Source: CAD feature listing. Evaluate the final solid. Frame: model axes, mm. A direction names the side the tool comes from. Give positions to 0.01 mm unless a question says otherwise; leave off trailing zeros. Order: outer loops, then holes, each group sorted by start corner. A loop starts at its lowest first (then second) coordinate and runs counter-clockwise, first axis right, second up. Notation, with made-up numbers: (66.5, 42) -> (94.5, 42) arc R18 ccw to (94.5, 69) -> close; hole circle Ø4 at (-11, 5.5). An arc over 180 degrees is marked (long way). Answer in a Markdown table with one row per item.
```python
from build123d import *

# Parameters (mm, degrees)
SKETCH1_R            = 2.675
BOSS_EXTRUDE6_DEPTH  = 10
BOSS_EXTRUDE8_START  = -21
BOSS_EXTRUDE8_DEPTH  = 21
SKETCH10_R           = 3.5
CUT_EXTRUDE5_DEPTH   = 191.966382811
SKETCH11_R           = 7.125
CUT_EXTRUDE6_DEPTH   = 5
CUT_EXTRUDE7_START   = -5
SKETCH12_R           = 7.125
CUT_EXTRUDE7_DEPTH   = 5
BOSS_EXTRUDE9_DEPTH  = 5
BOSS_EXTRUDE11_DEPTH = 12
BOSS_EXTRUDE13_START = 12
BOSS_EXTRUDE13_DEPTH = 12
SKETCH18_R           = 6.75
CUT_EXTRUDE11_DEPTH  = 1.67
CUT_EXTRUDE13_DEPTH  = 191.966382811
CUT_EXTRUDE14_DEPTH  = 191.966382811
CUT_EXTRUDE10_DEPTH  = 213.509902322
SKETCH26_R           = 2.675
BOSS_EXTRUDE14_DEPTH = 5
SKETCH27_R           = 2.675
BOSS_EXTRUDE15_DEPTH = 5
SKETCH30_R           = 2.675
CUT_EXTRUDE15_DEPTH  = 10
BOSS_EXTRUDE16_START = 1.67
SKETCH31_R           = 6.75
BOSS_EXTRUDE16_DEPTH = 1.67
SKETCH32_R           = 6.75
BOSS_EXTRUDE17_DEPTH = 2
SKETCH34_R           = 6.35
BOSS_EXTRUDE18_DEPTH = 1.5
SKETCH35_R           = 2.675
BOSS_EXTRUDE19_DEPTH = 4
CUT_EXTRUDE16_DEPTH  = 12
CUT_EXTRUDE17_DEPTH  = 12
FILLET1_R            = 10


with BuildPart() as part:
    # Sketch1 → Boss-Extrude6 (new body)
    with BuildSketch(Plane.XY):
        with BuildLine():
            Line((182.426294195, 92.707675116), (186.967804891, 79.877060143))
            ThreePointArc((186.967804891, 79.877060143), (187.827472336, 74.871963218), (186.967804891, 69.866866293))
            Line((186.967804891, 69.866866293), (182.426294195, 57.03625132))
            ThreePointArc((182.426294195, 57.03625132), (179.86789414, 53.655758914), (175.827472336, 52.371963218))
            Line((175.827472336, 52.371963218), (157.827472336, 52.371963218))
            Line((157.827472336, 52.371963218), (157.827472336, 64.371963218))
            Line((157.827472336, 64.371963218), (137.827472336, 64.371963218))
            Line((137.827472336, 64.371963218), (137.827472336, 85.371963218))
            Line((137.827472336, 85.371963218), (157.827472336, 85.371963218))
            Line((157.827472336, 85.371963218), (157.827472336, 97.371963218))
            Line((157.827472336, 97.371963218), (175.827472336, 97.371963218))
            ThreePointArc((175.827472336, 97.371963218), (179.86789414, 96.088167522), (182.426294195, 92.707675116))
        make_face()
        with Locations((155.487472336, 74.871963218)):
            Circle(SKETCH1_R, mode=Mode.SUBTRACT)
    extrude(amount=BOSS_EXTRUDE6_DEPTH)

    # Sketch9 → Boss-Extrude8 (add)
    with BuildSketch(Plane(origin=(0, 85.371963218, 0), x_dir=(1, 0, 0), z_dir=(0, 1, 0)).offset(BOSS_EXTRUDE8_START)):
        with BuildLine():
            Line((137.827472336, 0), (157.827472336, 0))
            ThreePointArc((157.827472336, 0), (154.893165251, 7.076438626), (147.81227561, 9.999988453))
            Line((147.81227561, 9.999988453), (137.827472336, 9.999988453))
            Line((137.827472336, 9.999988453), (137.827472336, 0))
        make_face()
    extrude(amount=BOSS_EXTRUDE8_DEPTH)

    # Sketch10 → Cut-Extrude5 (cut, through all)
    with BuildSketch(Plane(origin=(0, 85.371963218, 0), x_dir=(1, 0, 0), z_dir=(0, 1, 0))):
        with Locations(Location((147.827472336, 0, 0), (0, 0, 270))):
            Circle(SKETCH10_R)
    extrude(amount=-CUT_EXTRUDE5_DEPTH, mode=Mode.SUBTRACT)

    # Sketch11 → Cut-Extrude6 (cut)
    with BuildSketch(Plane(origin=(0, 85.371963218, 0), x_dir=(1, 0, 0), z_dir=(0, 1, 0))):
        with Locations(Location((147.827472336, 0, 0), (0, 0, 270))):
            Circle(SKETCH11_R)
    extrude(amount=-CUT_EXTRUDE6_DEPTH, mode=Mode.SUBTRACT)

    # Sketch12 → Cut-Extrude7 (cut)
    with BuildSketch(Plane.XZ.offset(-64.371963218).offset(CUT_EXTRUDE7_START)):
        with Locations(Location((147.827472336, 0, 0), (0, 0, 90))):
            Circle(SKETCH12_R)
    extrude(amount=CUT_EXTRUDE7_DEPTH, mode=Mode.SUBTRACT)

    # Sketch15 → Boss-Extrude9 (add)
    with BuildSketch(Plane.XY.offset(10)):
        Polygon((157.89790971, 79.046963218), (153.077034962, 79.046963218), (150.666597588, 74.871963218), (153.077034962, 70.696963218), (157.89790971, 70.696963218), (160.308347084, 74.871963218), align=None)
    extrude(amount=-BOSS_EXTRUDE9_DEPTH)

    # Sketch19 → Boss-Extrude11 (add)
    with BuildSketch(Plane(origin=(0, 85.371963218, 0), x_dir=(1, 0, 0), z_dir=(0, 1, 0))):
        with BuildLine():
            Line((157.827472336, -4.582575695), (157.827472336, -10))
            Line((157.827472336, -10), (152.410048031, -10))
            ThreePointArc((152.410048031, -10), (155.605646929, -7.778174593), (157.827472336, -4.582575695))
        make_face()
    extrude(amount=BOSS_EXTRUDE11_DEPTH)

    # Sketch21 → Boss-Extrude13 (add)
    with BuildSketch(Plane.XZ.offset(-64.371963218).offset(BOSS_EXTRUDE13_START)):
        with BuildLine():
            Line((157.827472336, 4.582575695), (157.827472336, 10))
            Line((157.827472336, 10), (152.410048031, 10))
            ThreePointArc((152.410048031, 10), (155.605646929, 7.778174593), (157.827472336, 4.582575695))
        make_face()
    extrude(amount=-BOSS_EXTRUDE13_DEPTH)

    # Sketch18 → Cut-Extrude11 (cut)
    with BuildSketch(Plane(origin=(0, 0, 0), x_dir=(-1, 0, 0), z_dir=(0, 0, -1))):
        with Locations((-173.633919606, 74.871963218)):
            Circle(SKETCH18_R)
    extrude(amount=-CUT_EXTRUDE11_DEPTH, mode=Mode.SUBTRACT)

    # Sketch23 → Cut-Extrude13 (cut, through all)
    with BuildSketch(Plane.XZ.offset(-64.371963218)):
        with BuildLine():
            Line((157.827472336, 4.582575695), (157.827472336, 0))
            Line((157.827472336, 0), (158.827472336, 0))
            ThreePointArc((158.827472336, 0), (158.574564966, 2.34520788), (157.827472336, 4.582575695))
        make_face()
    extrude(amount=CUT_EXTRUDE13_DEPTH, mode=Mode.SUBTRACT)

    # Sketch24 → Cut-Extrude14 (cut, through all)
    with BuildSketch(Plane(origin=(0, 85.371963218, 0), x_dir=(1, 0, 0), z_dir=(0, 1, 0))):
        with BuildLine():
            Line((157.827472336, -4.582575695), (157.827472336, 0))
            Line((157.827472336, 0), (158.827472336, 0))
            ThreePointArc((158.827472336, 0), (158.574564966, -2.34520788), (157.827472336, -4.582575695))
        make_face()
    extrude(amount=CUT_EXTRUDE14_DEPTH, mode=Mode.SUBTRACT)

    # Sketch14 → Cut-Extrude10 (cut, through all)
    with BuildSketch(Plane.XY.offset(10)):
        Polygon((157.89790971, 79.046963218), (153.077034962, 79.046963218), (150.666597588, 74.871963218), (153.077034962, 70.696963218), (157.89790971, 70.696963218), (160.308347084, 74.871963218), align=None)
    extrude(amount=-CUT_EXTRUDE10_DEPTH, mode=Mode.SUBTRACT)

    # Sketch26 → Boss-Extrude14 (add)
    with BuildSketch(Plane.XY.offset(10)):
        Polygon((153.077034962, 79.046963218), (150.666597588, 74.871963218), (153.077034962, 70.696963218), (157.89790971, 70.696963218), (160.308347084, 74.871963218), (157.89790971, 79.046963218), align=None)
        with Locations((155.487472336, 74.871963218)):
            Circle(SKETCH26_R, mode=Mode.SUBTRACT)
    extrude(amount=-BOSS_EXTRUDE14_DEPTH)

    # Sketch27 → Boss-Extrude15 (add)
    with BuildSketch(Plane.XY.offset(10)):
        with Locations((155.487472336, 74.871963218)):
            Circle(SKETCH27_R)
    extrude(amount=-BOSS_EXTRUDE15_DEPTH)

    # Sketch30 → Cut-Extrude15 (cut)
    with BuildSketch(Plane(origin=(0, 0, 5), x_dir=(-1, 0, 0), z_dir=(0, 0, -1))):
        with Locations((-155.487472336, 74.871963218)):
            Circle(SKETCH30_R)
    extrude(amount=-CUT_EXTRUDE15_DEPTH, mode=Mode.SUBTRACT)

    # Sketch31 → Boss-Extrude16 (add)
    with BuildSketch(Plane(origin=(0, 0, 1.67), x_dir=(-1, 0, 0), z_dir=(0, 0, -1)).offset(BOSS_EXTRUDE16_START)):
        with BuildLine():
            Line((-157.827472336, 85.371963218), (-158.827472336, 85.371963218))
            Line((-158.827472336, 85.371963218), (-158.827472336, 97.371963218))
            Line((-158.827472336, 97.371963218), (-175.827472336, 97.371963218))
            ThreePointArc((-175.827472336, 97.371963218), (-179.86789414, 96.088167522), (-182.426294195, 92.707675116))
            Line((-182.426294195, 92.707675116), (-186.967804891, 79.877060143))
            ThreePointArc((-186.967804891, 79.877060143), (-187.827472336, 74.871963218), (-186.967804891, 69.866866293))
            Line((-186.967804891, 69.866866293), (-182.426294195, 57.03625132))
            ThreePointArc((-182.426294195, 57.03625132), (-179.86789414, 53.655758914), (-175.827472336, 52.371963218))
            Line((-175.827472336, 52.371963218), (-158.827472336, 52.371963218))
            Line((-158.827472336, 52.371963218), (-158.827472336, 64.371963218))
            Line((-158.827472336, 64.371963218), (-157.827472336, 64.371963218))
            Line((-157.827472336, 64.371963218), (-157.827472336, 70.696963218))
            Line((-157.827472336, 70.696963218), (-157.89790971, 70.696963218))
            Line((-157.89790971, 70.696963218), (-160.308347084, 74.871963218))
            Line((-160.308347084, 74.871963218), (-157.89790971, 79.046963218))
            Line((-157.89790971, 79.046963218), (-157.827472336, 79.046963218))
            Line((-157.827472336, 79.046963218), (-157.827472336, 85.371963218))
        make_face()
        with Locations((-173.633919606, 74.871963218)):
            Circle(SKETCH31_R, mode=Mode.SUBTRACT)
    extrude(amount=-BOSS_EXTRUDE16_DEPTH)

    # Sketch32 → Boss-Extrude17 (add)
    with BuildSketch(Plane(origin=(0, 0, 0), x_dir=(-1, 0, 0), z_dir=(0, 0, -1))):
        with Locations((-173.633919606, 74.871963218)):
            Circle(SKETCH32_R)
    extrude(amount=-BOSS_EXTRUDE17_DEPTH)

    # Sketch34 → Boss-Extrude18 (add)
    with BuildSketch(Plane(origin=(0, 0, 0), x_dir=(-1, 0, 0), z_dir=(0, 0, -1))):
        with Locations(Location((-173.633919606, 74.871963218, 0), (0, 0, 180))):
            Circle(SKETCH34_R)
    extrude(amount=BOSS_EXTRUDE18_DEPTH)

    # Sketch35 → Boss-Extrude19 (add)
    with BuildSketch(Plane.XY.offset(10)):
        with BuildLine():
            Line((137.827472336, 85.371963218), (137.827472336, 64.371963218))
            Line((137.827472336, 64.371963218), (137.827472336, 52.371963218))
            Line((137.827472336, 52.371963218), (175.827472336, 52.371963218))
            ThreePointArc((175.827472336, 52.371963218), (179.86789414, 53.655758914), (182.426294195, 57.03625132))
            Line((182.426294195, 57.03625132), (186.967804891, 69.866866293))
            ThreePointArc((186.967804891, 69.866866293), (187.827472336, 74.871963218), (186.967804891, 79.877060143))
            Line((186.967804891, 79.877060143), (182.426294195, 92.707675116))
            ThreePointArc((182.426294195, 92.707675116), (179.86789414, 96.088167522), (175.827472336, 97.371963218))
            Line((175.827472336, 97.371963218), (137.827472336, 97.371963218))
            Line((137.827472336, 97.371963218), (137.827472336, 85.371963218))
        make_face()
        with Locations(Location((155.487472336, 74.871963218, 0), (0, 0, 180))):
            Circle(SKETCH35_R, mode=Mode.SUBTRACT)
    extrude(amount=BOSS_EXTRUDE19_DEPTH)

    # Sketch36 → Cut-Extrude16 (cut)
    with BuildSketch(Plane(origin=(0, 97.371963218, 0), x_dir=(1, 0, 0), z_dir=(0, 1, 0))):
        with BuildLine():
            Line((147.827472336, -11), (137.827472336, -11))
            Line((137.827472336, -11), (137.827472336, -10))
            Line((137.827472336, -10), (152.410048031, -10))
            ThreePointArc((152.410048031, -10), (150.172680216, -10.74709263), (147.827472336, -11))
        make_face()
    extrude(amount=-CUT_EXTRUDE16_DEPTH, mode=Mode.SUBTRACT)

    # Sketch38 → Cut-Extrude17 (cut)
    with BuildSketch(Plane.XZ.offset(-52.371963218)):
        with BuildLine():
            Line((147.827472336, 11), (137.827472336, 11))
            Line((137.827472336, 11), (137.827472336, 10))
            Line((137.827472336, 10), (152.410048031, 10))
            ThreePointArc((152.410048031, 10), (150.172680216, 10.74709263), (147.827472336, 11))
        make_face()
    extrude(amount=-CUT_EXTRUDE17_DEPTH, mode=Mode.SUBTRACT)

    # Fillet1
    # the kernel refuses this fillet: 10 mm, written as the material it takes off along each edge
    with BuildSketch(Plane(origin=(137.827472336, 39.371963218, -9.999988453), x_dir=(0.9999999999993333, 0, -1.1547030050344039e-06), z_dir=(0, 1, 0))) as fillet1_piece_1:
        with BuildLine():
            CenterArc((9.999988453, -10), FILLET1_R, 89.99993384, 90)
            Line((-1.1547e-05, -9.999988453), (-1.000011547, -9.999987298))
            Line((-1.000011547, -9.999987298), (-1, 1.155e-06))
            Line((-1, 1.155e-06), (1.155e-06, 1))
            ThreePointArc((1.155e-06, 1), (9.983284757, 0.999987318), (10.000001155, 1))
            Line((10.000001155, 1), (10, 0))
        make_face()
    extrude(amount=71, mode=Mode.SUBTRACT)


solid = part.part
```
(1) Section query C-C (y = 91.5). Return the cut outline in (x, z).
A:
| item | result |
|---|---|
| outline | (137.83, 11) -> (147.83, 11) arc R11 cw to (158.83, 0) -> (182.85, 0) -> (182.85, 14) -> (137.83, 14) -> close |
(2) Ray query, probe 1 along Z at (x, y) = (168.5, 83); probe 2 along X at (y, z) = (72, -0.25); probe 3 along Y at (x, z) = (141.5, 8.5). Return the intervals inside material, ascending.
A:
| item | result |
|---|---|
| probe 1 | z = 0 to 14 |
| probe 2 | x = 137.83 to 144.34, 151.32 to 152.32, 167.97 to 179.3 |
| probe 3 | y = 64.37 to 85.37 |
(3) Section query B-B (x = 146.5). Return the cut outline in (y, z).
A:
| item | result |
|---|---|
| outline | (52.37, 11) -> (64.37, 11) -> (64.37, 7) -> (69.37, 7) -> (69.37, 3.24) -> (80.37, 3.24) -> (80.37, 7) -> (85.37, 7) -> (85.37, 11) -> (97.37, 11) -> (97.37, 14) -> (52.37, 14) -> close; (64.37, -9.91) -> (85.37, -9.91) -> (85.37, -7) -> (80.37, -7) -> (80.37, -3.24) -> (69.37, -3.24) -> (69.37, -7) -> (64.37, -7) -> close |
(4) First-contact query: pin 1 Ø2.5 at (x, z) = (155, -1) entering from +Y; pin 2 Ø1.5 at (y, z) = (77.5, 8) entering from +X; pin 3 Ø1.5 at (x, z) = (182, 5.5) entering from -Y. Flat tips, straight axial feed; report the tip coordinate or a pass-through.
A:
| item | result |
|---|---|
| pin 1 | stops at y = 85.37 |
| pin 2 | stops at x = 187.71 |
| pin 3 | stops at y = 54.95 |
(5) Section query A-A (z = 12). Return the cut outline in (x, y) (3 decimals), plus the area to 3 significant figures.
A:
| item | result |
|---|---|
| outline | (137.827, 52.372) -> (175.827, 52.372) arc R7 ccw to (182.426, 57.036) -> (186.968, 69.867) arc R15 ccw to (186.968, 79.877) -> (182.426, 92.708) arc R7 ccw to (175.827, 97.372) -> (137.827, 97.372) -> close; hole circle Ø5.35 at (155.487, 74.872) |
| area | 2,080 mm^2 |
(6) Access query for faces 1 (the flat face through (148, 64.372, 8)), 2 (the flat face through (144.56, 69.372, -1.68)), 3 (the flat face through (166, 75, 0)). Directions: +Z, -Z, +X, -X, +Y, -Y. A direction counts if a zero-diameter tool reaches every point of the face in a straight line with its end or side. Return the directions, or none.
A:
| item | result |
|---|---|
| face 1 | -Z, -X, -Y |
| face 2 | -Y |
| face 3 | -Z |
(7) Pull-direction query (Z, two-part tool) for faces 4 (the flat face through (143, 91, 11)), 5 (the flat face through (151, 80.372, -2)), 6 (the flat face through (137.827, 75, 8)); classes: +Z half, -Z half, draft (parallel to the pull), parting line (faces both ways), or undercut.
A:
| item | result |
|---|---|
| face 4 | -Z half |
| face 5 | undercut |
| face 6 | draft |
